from build123d import *

# Parameters (mm, degrees)
SKETCH15_R          = 26
SKETCH15_R_2        = 21
BOSS_EXTRUDE2_DEPTH = 80
BOSS_EXTRUDE5_START = -10
SKETCH18_R          = 21
SKETCH18_R_2        = 16
BOSS_EXTRUDE5_DEPTH = 30
CHAMFER1_SIZE       = 5


with BuildPart() as part:
    # Sketch15 → Boss-Extrude2 (new body)
    with BuildSketch(Plane.XY):
        Circle(SKETCH15_R)
        Circle(SKETCH15_R_2, mode=Mode.SUBTRACT)
    extrude(amount=BOSS_EXTRUDE2_DEPTH)

    # Sketch18 → Boss-Extrude5 (add)
    with BuildSketch(Plane.XY.offset(80).offset(BOSS_EXTRUDE5_START)):
        Circle(SKETCH18_R)
        Circle(SKETCH18_R_2, mode=Mode.SUBTRACT)
    extrude(amount=BOSS_EXTRUDE5_DEPTH)

    # Chamfer1
    chamfer1_edges = [part.edges().sort_by_distance(p)[0] for p in [
        (-21, 0, 100),
    ]]
    chamfer(chamfer1_edges, length=CHAMFER1_SIZE - 0.0001)  # a hair under: the kernel refuses the full size


solid = part.part
The listing builds one solid part. Answer for the finished solid, in the listing's coordinates (mm). A direction names the side the tool comes from. Round coordinates to 2 decimals unless told otherwise and drop trailing zeros. Loops run counter-clockwise (first coordinate to the right, second up) from the corner with the lowest first, then second, coordinate; pieces in that order, holes last. Notation, with made-up numbers: M -24,76.25 L 21,76.25 A32 cw 21,108.25 Z; hole C 69.5,-20 d6. An arc over 180 degrees is marked long. Return JSON: item names as keys, results as strings.
Q1. Each of these flat-tipped pins is pushed along its axis until it touches: pin 1 Ø8 at (x, y) = (-16.5, -10.5) entering from -Z; pin 2 Ø8 at (x, z) = (-11, 23) entering from -Y; pin 3 Ø1.5 at (x, z) = (2, 22) entering from +Y; pin 4 Ø2 at (x, z) = (6, 14) entering from +Y. Where does it stop, or does it pass through?
Results list:
{"pin 1": "stops at z = 0", "pin 2": "stops at y = -25.04", "pin 3": "stops at y = 25.97", "pin 4": "stops at y = 25.51"}
Q2. Find section C-C, the plane z = 30.5. Determine the outline of the cut face in (x, y), plus the area to 3 significant figures.
Results list:
{"outline": "C 0,0 d52; hole C 0,0 d42", "area": "738 mm2"}
Q3. Which of the six approach directions +Z, -Z, +X, -X, +Y, -Y give full straight-line access (tool end or side, diameter ignored) to faces 5 (the face through (1.8, 21.3, 80)), 6 (the face through (-4.8, -15.5, 70)), 7 (the face through (-20.633, -15.821, 39.44))?
Results list:
{"face 5": "+Z", "face 6": "-Z", "face 7": "+Z, -Z"}
Q4. The mould has two halves that part along Y. Classify faces 1 (the face through (20.03, 6.31, 87.4)), 2 (the face through (20.03, 6.31, 34.51)), 3 (the face through (1.8, 21.3, 0)), 4 (the face through (-3.47, -15.62, 84.79)): released by +Y, released by -Y, zero draft, split by the parting line, or undercut.
Results list:
{"face 1": "split by the parting line", "face 2": "undercut", "face 3": "zero draft", "face 4": "undercut"}
Q5. Find the intervals of material crossed by line 1 along Y through (x, z) = (0, 35); line 2 along Y through (x, z) = (0, 84.75); line 3 along Z through (x, y) = (18, 12), in increasing order. Write a range as from..to.
Results list:
{"line 1": "y = -26..-21, 21..26", "line 2": "y = -21..-16, 16..21", "line 3": "z = 0..80"}
Q6. Find section D-D, the plane z = 84.5. Determine the outline of the cut face in (x, y).
Results list:
{"outline": "C 0,0 d42; hole C 0,0 d32"}
